from build123d import *

# Parameters (mm, degrees)
ESQUISSE1_R             = 7.6
BOSS_EXTRU_1_DEPTH      = 25
ESQUISSE3_R             = 7.6
ESQUISSE3_R_2           = 4.4
BOSS_EXTRU_3_DEPTH      = 2.5
BOSS_EXTRU_3_2_DEPTH    = 2.5
BOSS_EXTRU_5_START      = -2.5
ESQUISSE1_4_R           = 7.6
BOSS_EXTRU_5_DEPTH      = 2.5
ESQUISSE7_R             = 19.75
ESQUISSE7_R_2           = 1.7
ESQUISSE7_R_3           = 10.25
ENL_V_MAT_EXTRU_1_DEPTH = 14
BOSS_EXTRU_9_START      = -3
BOSS_EXTRU_9_DEPTH      = 3
ESQUISSE7_4_R           = 1.7
ENL_V_MAT_EXTRU_2_DEPTH = 52.87063246
ENL_V_START             = -24
ESQUISSE11_R            = 7.6
ESQUISSE11_R_2          = 7.7
ENL_V_MAT_EXTRU_3_DEPTH = 24
CONG_2_R                = 2


with BuildPart() as part:
    # Esquisse1 → Boss.-Extru.1 (new body)
    with BuildSketch(Plane(origin=(0, 0, 0), x_dir=(1, 0, 0), z_dir=(0, 1, 0))):
        Polygon((-26, -21), (26, -21), (38, -21), (42, -17), (42, 0), (42, 8), (38, 12), (24, 12), (20, 8), (20, 1), (20, -4), (17, -4), (-17, -4), (-20, -4), (-20, 1), (-20, 8), (-24, 12), (-38, 12), (-42, 8), (-42, 0), (-42, -17), (-38, -21), align=None)
        with Locations(Location((-30, 0, 0), (0, 0, 270))):
            Circle(ESQUISSE1_R, mode=Mode.SUBTRACT)
        with Locations(Location((30, 0, 0), (0, 0, 90))):
            Circle(ESQUISSE1_R, mode=Mode.SUBTRACT)
    extrude(amount=BOSS_EXTRU_1_DEPTH)


with BuildPart() as body_2:
    # Esquisse3 → Boss.-Extru.3 (new body)
    with BuildSketch(Plane.XZ):
        with Locations(Location((-30, 0, 0), (0, 0, 90))):
            Circle(ESQUISSE3_R)
        with Locations(Location((-30, 0, 0), (0, 0, 270))):
            Circle(ESQUISSE3_R_2, mode=Mode.SUBTRACT)
    extrude(amount=BOSS_EXTRU_3_DEPTH)


with BuildPart() as body_3:
    # Esquisse3 → Boss.-Extru.3 2 (new body)
    with BuildSketch(Plane.XZ):
        with Locations(Location((30, 0, 0), (0, 0, 270))):
            Circle(ESQUISSE3_R)
        with Locations(Location((30, 0, 0), (0, 0, 90))):
            Circle(ESQUISSE3_R_2, mode=Mode.SUBTRACT)
    extrude(amount=BOSS_EXTRU_3_2_DEPTH)


with BuildPart() as boss_extru_5_tool:
    # Esquisse1<4> → Boss.-Extru.5 (new body)
    with BuildSketch(Plane(origin=(0, 0, 0), x_dir=(1, 0, 0), z_dir=(0, 1, 0)).offset(BOSS_EXTRU_5_START)):
        Polygon((-26, -21), (26, -21), (38, -21), (42, -17), (42, 0), (42, 8), (38, 12), (24, 12), (20, 8), (20, 1), (20, -4), (17, -4), (-17, -4), (-20, -4), (-20, 1), (-20, 8), (-24, 12), (-38, 12), (-42, 8), (-42, 0), (-42, -17), (-38, -21), align=None)
        with Locations(Location((-30, 0, 0), (0, 0, 90))):
            Circle(ESQUISSE1_4_R, mode=Mode.SUBTRACT)
        with Locations(Location((30, 0, 0), (0, 0, 90))):
            Circle(ESQUISSE1_4_R, mode=Mode.SUBTRACT)
    extrude(amount=BOSS_EXTRU_5_DEPTH)


with BuildPart() as part_1:
    add(part.part)


with BuildPart() as part_2:
    # Boss.-Extru.5: joined with boss_extru_5_tool
    add(part_1.part.fuse(boss_extru_5_tool.part, body_2.part, body_3.part, tol=0.00001))

    # Congé1
    # a fillet whose section is not a circle: 4 mm, written as the material it takes off along each edge
    with BuildSketch(Plane(origin=(-42, 29.142135624, 17), x_dir=(0, 0, -1), z_dir=(0, -1, 0)), Plane(origin=(-38, -6.642135624, -12), x_dir=(-0.707106781186547, 0, 0.7071067811865481), z_dir=(0, 1, 0)), Plane(origin=(-24, -6.642135624, -12), x_dir=(-1, 0, 0), z_dir=(0, 1, 0)), Plane(origin=(-20, -6.642135624, -8), x_dir=(-0.707106781186547, 0, -0.7071067811865481), z_dir=(0, 1, 0)), Plane(origin=(42, -6.642135624, 17), x_dir=(0, 0, -1), z_dir=(0, 1, 0)), Plane(origin=(42, -6.642135624, -8), x_dir=(-0.7071067811865487, 0, -0.7071067811865465), z_dir=(0, 1, 0)), Plane(origin=(38, -6.642135624, -12), x_dir=(-1, 0, 0), z_dir=(0, 1, 0)), Plane(origin=(24, -6.642135624, -12), x_dir=(-0.7071067811865459, 0, 0.7071067811865491), z_dir=(0, 1, 0)), Plane(origin=(20, -6.642135624, -8), x_dir=(0, 0, 1), z_dir=(0, 1, 0))) as cong_1_piece_1:
        with BuildLine():
            add(Edge.make_bspline([(1.656854249, 0), (1.35356905, 0), (1.050283851, 0), (0.373674798, 0.056927592), (-0.223974097, 0.30448187), (-0.742662833, 0.742662833), (-0.957117854, 0.957117854), (-1.171572875, 1.171572875)], knots=[0, 0, 0, 0, 0, 0, 0.5, 0.5, 1, 1, 1, 1, 1, 1], degree=5))
            Line((-1.171572875, 1.171572875), (0, 0))
            Line((0, 0), (1.656854249, 0))
        make_face()
    extrude(amount=35.784271247, mode=Mode.SUBTRACT)
    with BuildSketch(Plane(origin=(-42, 29.142135624, -8), x_dir=(0, 0, 1), z_dir=(0, -1, 0)), Plane(origin=(-38, 29.142135624, 21), x_dir=(1, 0, 0), z_dir=(0, -1, 0)), Plane(origin=(38, -6.642135624, 21), x_dir=(-1, 0, 0), z_dir=(0, 1, 0))) as cong_1_piece_2:
        with BuildLine():
            add(Edge.make_bspline([(1.656854249, 0), (1.35356905, 0), (1.050283851, 0), (0.373674798, -0.056927592), (-0.223974097, -0.30448187), (-0.742662833, -0.742662833), (-0.957117854, -0.957117854), (-1.171572875, -1.171572875)], knots=[0, 0, 0, 0, 0, 0, 0.5, 0.5, 1, 1, 1, 1, 1, 1], degree=5))
            Line((-1.171572875, -1.171572875), (0, 0))
            Line((0, 0), (1.656854249, 0))
        make_face()
    extrude(amount=35.784271247, mode=Mode.SUBTRACT)

    # Esquisse7 → Enlèv. mat.-Extru.1 (cut)
    with BuildSketch(Plane(origin=(0, 0, 4), x_dir=(-1, 0, 0), z_dir=(0, 0, -1))):
        with Locations((0, -5.5)):
            Circle(ESQUISSE7_R)
        with Locations((-14.488887394, -1.617714323)):
            Circle(ESQUISSE7_R_2, mode=Mode.SUBTRACT)
        with Locations((10.606601718, 5.106601718)):
            Circle(ESQUISSE7_R_2, mode=Mode.SUBTRACT)
        with Locations((3.882285677, -19.988887394)):
            Circle(ESQUISSE7_R_2, mode=Mode.SUBTRACT)
        with Locations((0, -5.5)):
            Circle(ESQUISSE7_R_3, mode=Mode.SUBTRACT)
        with Locations((-9.899494937, -15.399494937)):
            Circle(ESQUISSE7_R_2, mode=Mode.SUBTRACT)
    extrude(amount=-ENL_V_MAT_EXTRU_1_DEPTH, mode=Mode.SUBTRACT)

    # Esquisse10 → Boss.-Extru.9 (add)
    with BuildSketch(Plane.XY.offset(21).offset(BOSS_EXTRU_9_START)):
        with BuildLine():
            Line((19.520822216, -2.5), (-19.520822216, -2.5))
            ThreePointArc((-19.520822216, -2.5), (0, -25.25), (19.520822216, -2.5))
        make_face()
    extrude(amount=BOSS_EXTRU_9_DEPTH)

    # Esquisse7<4> → Enlèv. mat.-Extru.2 (cut, through all)
    with BuildSketch(Plane(origin=(0, 0, 4), x_dir=(-1, 0, 0), z_dir=(0, 0, -1))):
        with Locations((3.882285677, -19.988887394)):
            Circle(ESQUISSE7_4_R)
        with Locations((-14.488887394, -1.617714323)):
            Circle(ESQUISSE7_4_R)
        with Locations((10.606601718, 5.106601718)):
            Circle(ESQUISSE7_4_R)
        with BuildLine():
            Line((-9.801147892, -2.5), (9.801147892, -2.5))
            ThreePointArc((9.801147892, -2.5), (0, 4.75), (-9.801147892, -2.5))
        make_face()
        with BuildLine():
            ThreePointArc((10.25, -5.5), (10.137165923, -3.983303902), (9.801147892, -2.5))
            Line((9.801147892, -2.5), (-9.801147892, -2.5))
            ThreePointArc((-9.801147892, -2.5), (-1.516696098, -15.637165923), (10.25, -5.5))
        make_face()
    extrude(amount=-ENL_V_MAT_EXTRU_2_DEPTH, mode=Mode.SUBTRACT)

    # Esquisse11 → Enlèv. mat.-Extru.3 (cut)
    with BuildSketch(Plane(origin=(0, 25, 0), x_dir=(1, 0, 0), z_dir=(0, 1, 0)).offset(ENL_V_START)):
        with Locations(Location((-30, 0, 0), (0, 0, 90))):
            Circle(ESQUISSE11_R)
        with Locations(Location((30, 0, 0), (0, 0, 270))):
            Circle(ESQUISSE11_R_2)
    extrude(amount=ENL_V_MAT_EXTRU_3_DEPTH, mode=Mode.SUBTRACT)

    # Congé2
    cong_2_edges = [part_2.edges().sort_by_distance(p)[0] for p in [
        (-19.520822216, -2.5, 19.5),
        (19.520822216, -2.5, 19.5),
    ]]
    fillet(cong_2_edges, radius=CONG_2_R)


solid = part_2.part
CAD build for the part. Positions are in the model's coordinates, mm. A direction names the side the tool comes from. Coordinates: 2 decimals unless noted, no trailing zeros. Loops run counter-clockwise (first coordinate to the right, second up) from the corner with the lowest first, then second, coordinate; pieces in that order, holes last. Notation, with made-up numbers: (31, -20.5) - (38, -20.5) arc R12 ccw to (38, -0.5) - close; hole circle Ø5 at (-27.5, 18). An arc over 180 degrees is marked (long way). Write item = value, one per line. Start each with the question number.
Q1. Cut at B-B, the plane x = 30. List the corners of the cut face in (y, z).
Q2. Cut at C-C, the plane y = -12. List the corners of the cut face in (x, z).
Q3. Flat gauge pins, fed straight in: pin 1 Ø8 at (x, y) = (24.5, -13) entering from +Z; pin 2 Ø1 at (x, y) = (-10.5, 0.5) entering from -Z; pin 3 Ø8 at (x, z) = (-21.5, 16.5) entering from -Y; pin 4 Ø11.5 at (x, z) = (-30, 0) entering from +Y. Where does each tip first touch, or does it go through?
Q4. Drill centre lines: L1, parallel to X at y = -1.3, z = 0; L2, parallel to X at y = 15, z = 0; L3, parallel to Z at x = 30, y = -0.6. Where is each one in solid material? Low to high.
Q5. Which spindle directions (+Z, -Z, +X, -X, +Y, -Y) get a long thin tool onto all of the face, cutting with end or side? Do faces 1 (the flat face through (-20, 11, -1)), 2 (the cylindrical face through (22.483, 12.832, -1.669)), 3 (the cylindrical face through (-0.392, 14.246, 10.902)). Say none if no direction does.
Q6. Cut at D-D, the plane z = 14. List the corners of the cut face in (x, y).
Q7. Pull direction Z, two halves, no side cores. Call faces 4 (the cylindrical face through (23.6, 0.5, -4.1)), 5 (the cylindrical face through (-0.447, -25.245, 19.479)), 6 (the flat face through (-40, 11, 19)), 7 (the flat face through (22, 11, -10)): pulls with the +Z half, pulls with the -Z half, needs draft (parallel to the pull), parting line crosses it, or undercut.
Q8. Cut at A-A, the plane z = 0. List the corners of the cut face in (x, y).
Computed:
q1.outline = (-2.5, -12) - (25, -12) - (25, -7.7) - (1, -7.7) - (1, -7.6) - (0, -7.6) - (0, -4.4) - (-2.5, -4.4) - close; (-2.5, 4.4) - (0, 4.4) - (0, 7.6) - (1, 7.6) - (1, 7.7) - (25, 7.7) - (25, 21) - (-2.5, 21) - close
q2.outline = (-18.65, 18) - (-7.93, 18) - (-7.93, 21) - (-18.65, 21) - close; (7.93, 18) - (18.65, 18) - (18.65, 21) - (7.93, 21) - close
q3.pin_1 = through
q3.pin_2 = 18
q3.pin_3 = -14.07
q3.pin_4 = 0
q4.L1 = -42 to -34.4, -25.6 to -20, 20 to 25.6, 34.4 to 42
q4.L2 = -42 to -37.6, -22.4 to -20, 20 to 22.3, 37.7 to 42
q4.L3 = -12 to -4.4, 4.4 to 21
q5.face_1 = -Z, +Y, -Y
q5.face_2 = +Y
q5.face_3 = -Z, -Y
q6.outline = (-42, -2.5) - (-19.52, -2.5) arc R19.75 cw to (19.52, -2.5) - (42, -2.5) - (42, 25) - (-42, 25) - close
q7.face_4 = undercut
q7.face_5 = needs draft
q7.face_6 = pulls with the +Z half
q7.face_7 = pulls with the -Z half
q8.outline = (-42, -2.5) - (-34.4, -2.5) - (-34.4, 0) - (-37.6, 0) - (-37.6, 25) - (-42, 25) - close; (-25.6, -2.5) - (-20, -2.5) - (-20, 25) - (-22.4, 25) - (-22.4, 0) - (-25.6, 0) - close; (20, -2.5) - (25.6, -2.5) - (25.6, 0) - (22.4, 0) - (22.4, 1) - (22.3, 1) - (22.3, 25) - (20, 25) - close; (34.4, -2.5) - (42, -2.5) - (42, 25) - (37.7, 25) - (37.7, 1) - (37.6, 1) - (37.6, 0) - (34.4, 0) - close
